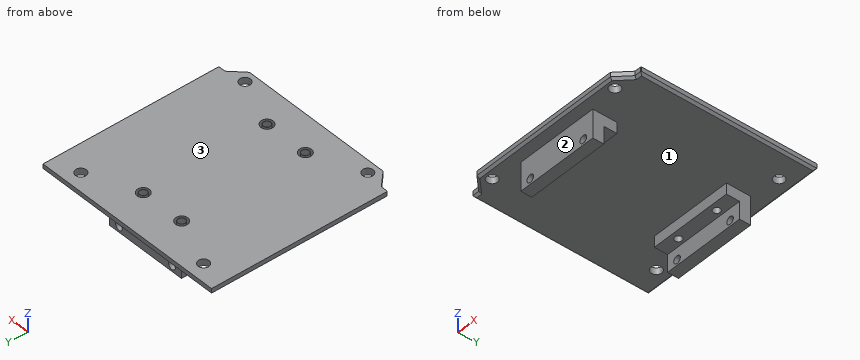
from build123d import *

# Parameters (mm, degrees)
SKETCH3_W             = 38
SKETCH3_H             = 6
BOSS_EXTRUDE2_DEPTH   = 8
BOSS_EXTRUDE2_2_DEPTH = 8
SKETCH1_R             = 2.43
BOSS_EXTRUDE3_DEPTH   = 3
CHAMFER1_SIZE         = 1
SKETCH4_W             = 38
SKETCH4_H             = 5
BOSS_EXTRUDE4_DEPTH   = 16
SKETCH5_R             = 1.75
CUT_EXTRUDE1_DEPTH    = 80
SKETCH6_R             = 1.625
CUT_EXTRUDE2_DEPTH    = 10
SKETCH7_R             = 2.75
SKETCH7_R_2           = 1.75
CUT_EXTRUDE3_DEPTH    = 4


with BuildPart() as part:
    # Sketch3 → Boss-Extrude2 (new body)
    with BuildSketch(Plane.XY):
        with Locations((152.499981225, 110.845805079)):
            Rectangle(SKETCH3_W, SKETCH3_H)
    extrude(amount=-BOSS_EXTRUDE2_DEPTH)



with BuildPart() as body_2:
    # Sketch3 → Boss-Extrude2 2 (new body)
    with BuildSketch(Plane.XY):
        with Locations((152.499981225, 166.845805079)):
            Rectangle(SKETCH3_W, SKETCH3_H)
    extrude(amount=-BOSS_EXTRUDE2_2_DEPTH)


with BuildPart() as body_3:
    # Sketch1 → Boss-Extrude3 (new body)
    with BuildSketch(Plane.XY):
        Polygon((197.000000954, 103.088447924), (197.000000954, 183.154169798), (107.999998748, 183.154169798), (107.999998748, 103.08845101), (108.242627497, 102.845828652), (111.242642284, 102.845828652), (117.242639543, 96.845823944), (187.757360159, 96.845823944), (193.757357418, 102.845828652), (196.757376569, 102.845828652), align=None)
        with Locations((184.906666899, 176.322621726)):
            Circle(SKETCH1_R, mode=Mode.SUBTRACT)
        with Locations((120.09, 176.322621726)):
            Circle(SKETCH1_R, mode=Mode.SUBTRACT)
        with Locations((184.906666899, 101.371103796)):
            Circle(SKETCH1_R, mode=Mode.SUBTRACT)
        with Locations((120.09, 101.371103796)):
            Circle(SKETCH1_R, mode=Mode.SUBTRACT)
    extrude(amount=-BOSS_EXTRUDE3_DEPTH)

    # Chamfer1
    # the kernel refuses this chamfer: 1 mm, written as the material it takes off along each edge
    with BuildSketch(Plane(origin=(105.670944509, 102.845828652, -3), x_dir=(0, -0.027495876610582174, 0.9996219169112968), z_dir=(1, 0, 0))) as chamfer1_piece_1_section:
        Polygon((CHAMFER1_SIZE * 0.999621916911, -CHAMFER1_SIZE * 0.0274958766106), (-CHAMFER1_SIZE * 0.0274958766106, -CHAMFER1_SIZE * 0.999621916911), (0, 0), align=None)
    chamfer1_piece_1 = extrude(amount=8.143380763, mode=Mode.PRIVATE)
    chamfer1_piece_1 = split(chamfer1_piece_1, bisect_by=Plane(origin=(109.611460338, 104.477012624, -2.663729969), z_dir=(-0.7071072202160112, -0.7071063421568112, 0)), keep=Keep.TOP, mode=Mode.PRIVATE)
    add(chamfer1_piece_1, mode=Mode.SUBTRACT)
    with BuildSketch(Plane(origin=(109.424188934, 104.664284261, -3), x_dir=(-0.019442532877514053, -0.01944250873450663, 0.9996219169112968), z_dir=(0.7071063421568113, -0.7071072202160114, 0))) as chamfer1_piece_2_section:
        Polygon((CHAMFER1_SIZE * 0.999621916911, -CHAMFER1_SIZE * 0.0274958766106), (-CHAMFER1_SIZE * 0.0274958766106, -CHAMFER1_SIZE * 0.999621916911), (0, 0), align=None)
    chamfer1_piece_2 = extrude(amount=13.628648741, mode=Mode.PRIVATE)
    chamfer1_piece_2 = split(chamfer1_piece_2, bisect_by=Plane(origin=(115.495387611, 102.845828652, -2.667041635), z_dir=(0, -1, 0)), keep=Keep.TOP, mode=Mode.PRIVATE)
    add(chamfer1_piece_2, mode=Mode.SUBTRACT)
    with BuildSketch(Plane(origin=(191.18567443, 102.845828652, -3), x_dir=(0, -0.027495876610582174, 0.9996219169112968), z_dir=(1, 0, 0))) as chamfer1_piece_3_section:
        Polygon((CHAMFER1_SIZE * 0.999621916911, -CHAMFER1_SIZE * 0.0274958766106), (-CHAMFER1_SIZE * 0.0274958766106, -CHAMFER1_SIZE * 0.999621916911), (0, 0), align=None)
    chamfer1_piece_3 = extrude(amount=8.143385128, mode=Mode.PRIVATE)
    chamfer1_piece_3 = split(chamfer1_piece_3, bisect_by=Plane(origin=(195.388540462, 104.477013723, -2.663729975), z_dir=(0.7071072202160112, -0.7071063421568112, 0)), keep=Keep.TOP, mode=Mode.PRIVATE)
    add(chamfer1_piece_3, mode=Mode.SUBTRACT)
    with BuildSketch(Plane(origin=(185.938906809, 95.027368335, -3), x_dir=(0.019442532877507145, -0.019442508734499722, 0.999621916911297), z_dir=(0.7071063421568113, 0.7071072202160114, 0))) as chamfer1_piece_4_section:
        Polygon((CHAMFER1_SIZE * 0.999621916911, -CHAMFER1_SIZE * 0.0274958766106), (-CHAMFER1_SIZE * 0.0274958766106, -CHAMFER1_SIZE * 0.999621916911), (0, 0), align=None)
    chamfer1_piece_4 = extrude(amount=13.628648741, mode=Mode.PRIVATE)
    chamfer1_piece_4 = split(chamfer1_piece_4, bisect_by=Plane(origin=(189.504612091, 102.845828652, -2.667041635), z_dir=(0, -1, 0)), keep=Keep.TOP, mode=Mode.PRIVATE)
    add(chamfer1_piece_4, mode=Mode.SUBTRACT)
    with BuildSketch(Plane(origin=(114.670956555, 96.845823944, -3), x_dir=(0, -0.027495876610582174, 0.9996219169112968), z_dir=(1, 0, 0))) as chamfer1_piece_5:
        Polygon((CHAMFER1_SIZE * 0.999621916911, -CHAMFER1_SIZE * 0.0274958766106), (-CHAMFER1_SIZE * 0.0274958766106, -CHAMFER1_SIZE * 0.999621916911), (0, 0), align=None)
    extrude(amount=75.658086593, mode=Mode.SUBTRACT)
    with BuildSketch(Plane(origin=(107.999998748, 185.725852786, -3), x_dir=(-0.027495876610582174, 0, 0.9996219169112968), z_dir=(0, -1, 0))) as chamfer1_piece_6:
        Polygon((CHAMFER1_SIZE * 0.999621916911, -CHAMFER1_SIZE * 0.0274958766106), (-CHAMFER1_SIZE * 0.0274958766106, -CHAMFER1_SIZE * 0.999621916911), (0, 0), align=None)
    extrude(amount=85.209084764, mode=Mode.SUBTRACT)
    with BuildSketch(Plane(origin=(199.571683942, 183.154169798, -3), x_dir=(0, 0.027495876610582174, 0.9996219169112968), z_dir=(-1, 0, 0))) as chamfer1_piece_7:
        Polygon((CHAMFER1_SIZE * 0.999621916911, -CHAMFER1_SIZE * 0.0274958766106), (-CHAMFER1_SIZE * 0.0274958766106, -CHAMFER1_SIZE * 0.999621916911), (0, 0), align=None)
    extrude(amount=94.143368181, mode=Mode.SUBTRACT)
    with BuildSketch(Plane(origin=(197.000000954, 100.516764936, -3), x_dir=(0.027495876610582174, 0, 0.9996219169112968), z_dir=(0, 1, 0))) as chamfer1_piece_8:
        Polygon((CHAMFER1_SIZE * 0.999621916911, -CHAMFER1_SIZE * 0.0274958766106), (-CHAMFER1_SIZE * 0.0274958766106, -CHAMFER1_SIZE * 0.999621916911), (0, 0), align=None)
    extrude(amount=85.20908785, mode=Mode.SUBTRACT)
    with BuildSketch(Plane(origin=(105.670944509, 102.845828652, -3), x_dir=(0, -0.027495876610582174, 0.9996219169112968), z_dir=(1, 0, 0))) as chamfer1_piece_9a_section:
        Polygon((CHAMFER1_SIZE * 0.999621916911, -CHAMFER1_SIZE * 0.0274958766106), (-CHAMFER1_SIZE * 0.0274958766106, -CHAMFER1_SIZE * 0.999621916911), (0, 0), align=None)
    chamfer1_piece_9a = extrude(amount=8.143380763, mode=Mode.PRIVATE)
    chamfer1_piece_9a = split(chamfer1_piece_9a, bisect_by=Plane(origin=(111.621802536, 102.46666793, -2.681906862), z_dir=(0.7071072202160112, 0.7071063421568112, 0)), keep=Keep.TOP, mode=Mode.PRIVATE)
    with BuildSketch(Plane(origin=(109.424188934, 104.664284261, -3), x_dir=(-0.019442532877514053, -0.01944250873450663, 0.9996219169112968), z_dir=(0.7071063421568113, -0.7071072202160114, 0))) as chamfer1_piece_9b_section:
        Polygon((CHAMFER1_SIZE * 0.999621916911, -CHAMFER1_SIZE * 0.0274958766106), (-CHAMFER1_SIZE * 0.0274958766106, -CHAMFER1_SIZE * 0.999621916911), (0, 0), align=None)
    chamfer1_piece_9b = extrude(amount=13.628648741, mode=Mode.PRIVATE)
    chamfer1_piece_9b = split(chamfer1_piece_9b, bisect_by=Plane(origin=(110.706428382, 102.845828652, -2.681906862), z_dir=(0, 1, 0)), keep=Keep.TOP, mode=Mode.PRIVATE)
    chamfer1_piece_9 = chamfer1_piece_9a & chamfer1_piece_9b
    add(chamfer1_piece_9, mode=Mode.SUBTRACT)
    with BuildSketch(Plane(origin=(185.938906809, 95.027368335, -3), x_dir=(0.019442532877507145, -0.019442508734499722, 0.999621916911297), z_dir=(0.7071063421568113, 0.7071072202160114, 0))) as chamfer1_piece_10a_section:
        Polygon((CHAMFER1_SIZE * 0.999621916911, -CHAMFER1_SIZE * 0.0274958766106), (-CHAMFER1_SIZE * 0.0274958766106, -CHAMFER1_SIZE * 0.999621916911), (0, 0), align=None)
    chamfer1_piece_10a = extrude(amount=13.628648741, mode=Mode.PRIVATE)
    chamfer1_piece_10a = split(chamfer1_piece_10a, bisect_by=Plane(origin=(194.29357132, 102.845828652, -2.681906862), z_dir=(0, 1, 0)), keep=Keep.TOP, mode=Mode.PRIVATE)
    with BuildSketch(Plane(origin=(191.18567443, 102.845828652, -3), x_dir=(0, -0.027495876610582174, 0.9996219169112968), z_dir=(1, 0, 0))) as chamfer1_piece_10b_section:
        Polygon((CHAMFER1_SIZE * 0.999621916911, -CHAMFER1_SIZE * 0.0274958766106), (-CHAMFER1_SIZE * 0.0274958766106, -CHAMFER1_SIZE * 0.999621916911), (0, 0), align=None)
    chamfer1_piece_10b = extrude(amount=8.143385128, mode=Mode.PRIVATE)
    chamfer1_piece_10b = split(chamfer1_piece_10b, bisect_by=Plane(origin=(193.378197166, 102.46666793, -2.681906862), z_dir=(-0.7071072202160112, 0.7071063421568112, 0)), keep=Keep.TOP, mode=Mode.PRIVATE)
    chamfer1_piece_10 = chamfer1_piece_10a & chamfer1_piece_10b
    add(chamfer1_piece_10, mode=Mode.SUBTRACT)


with BuildPart() as part_1:
    add(part.part)

    add(body_2.part)  # Boss-Extrude4 merges body 2

    add(body_3.part)  # Boss-Extrude4 merges body 3
    # Sketch4 → Boss-Extrude4 (add)
    with BuildSketch(Plane.XY):
        with Locations((152.499981225, 172.345805079)):
            Rectangle(SKETCH4_W, SKETCH4_H)
        with Locations((152.499981225, 105.345805079)):
            Rectangle(SKETCH4_W, SKETCH4_H)
    extrude(amount=-BOSS_EXTRUDE4_DEPTH)

    # Sketch5 → Cut-Extrude1 (cut)
    with BuildSketch(Plane(origin=(0, 102.845805079, 0), x_dir=(-1, 0, 0), z_dir=(0, -1, 0))):
        with Locations(Location((-166.499981225, 13.4, 0), (0, 0, 180))):
            Circle(SKETCH5_R)
        with Locations(Location((-138.499981225, 13.4, 0), (0, 0, 180))):
            Circle(SKETCH5_R)
    extrude(amount=-CUT_EXTRUDE1_DEPTH, mode=Mode.SUBTRACT)

    # Sketch6 → Cut-Extrude2 (cut)
    with BuildSketch(Plane(origin=(0, 0, -8), x_dir=(-1, 0, 0), z_dir=(0, 0, -1))):
        with Locations((-162.624981225, 110.595805079)):
            Circle(SKETCH6_R)
        with Locations((-142.374981225, 110.595805079)):
            Circle(SKETCH6_R)
        with Locations((-162.624981225, 167.095805079)):
            Circle(SKETCH6_R)
        with Locations((-142.374981225, 167.095805079)):
            Circle(SKETCH6_R)
    extrude(amount=-CUT_EXTRUDE2_DEPTH, mode=Mode.SUBTRACT)

    # Sketch7 → Cut-Extrude3 (cut)
    # profile 1 of 4: a face of its own
    with BuildSketch(Plane.XY):
        with Locations((162.624981225, 167.095805079)):
            Circle(SKETCH7_R)
        with Locations((162.624981225, 167.095805079)):
            Circle(SKETCH7_R_2, mode=Mode.SUBTRACT)
    # profile 2 of 4: a face of its own
    with BuildSketch(Plane.XY):
        with Locations((142.374981225, 167.095805079)):
            Circle(SKETCH7_R)
        with Locations((142.374981225, 167.095805079)):
            Circle(SKETCH7_R_2, mode=Mode.SUBTRACT)
    # profile 3 of 4: a face of its own
    with BuildSketch(Plane.XY):
        with Locations((162.624981225, 110.595805079)):
            Circle(SKETCH7_R)
        with Locations((162.624981225, 110.595805079)):
            Circle(SKETCH7_R_2, mode=Mode.SUBTRACT)
    # profile 4 of 4: a face of its own
    with BuildSketch(Plane.XY):
        with Locations((142.374981225, 110.595805079)):
            Circle(SKETCH7_R)
        with Locations((142.374981225, 110.595805079)):
            Circle(SKETCH7_R_2, mode=Mode.SUBTRACT)
    extrude(amount=-CUT_EXTRUDE3_DEPTH, mode=Mode.SUBTRACT)


solid = part_1.part
Check sheet for the modelled part. Datum: model origin and axes. Units: mm. Face numbers are marked on the shaded views. Coordinates: 2 decimals unless noted, no trailing zeros. Write each loop counter-clockwise with the first axis right and the second up, starting at its lowest first coordinate (ties: lowest second). Pieces come first, ordered by that corner, then holes.
Item 1: Scan lines: probe 1 along Y at (x, z) = (120.09, -1.9); probe 2 along Y at (x, z) = (168, -6.25); probe 3 along Y at (x, z) = (160, -12.5). Record each from-to range of solid material in increasing order.
Numbers:
probe 1: y = 96.85 to 98.94, 103.8 to 173.89, 178.75 to 183.15
probe 2: y = 102.85 to 113.85, 163.85 to 174.85
probe 3: y = 102.85 to 107.85, 169.85 to 174.85
Item 2: Depth check by flat-ended pin: pin 1 Ø4 at (x, y) = (120.09, 176.32) entering from +Z; pin 2 Ø3 at (x, y) = (150.5, 112.5) entering from -Z; pin 3 Ø1.5 at (x, z) = (161.5, -6.5) entering from +Y; pin 4 Ø5 at (x, y) = (162.62, 167.1) entering from +Z. Enter the tip coordinate at first touch or a pass-through.
Numbers:
pin 1: passes through
pin 2: stops at z = -8
pin 3: stops at y = 174.85
pin 4: stops at z = 0
Item 3: Cross-section at B-B on x = 120.09. Record the boundary of the cut face in (y, z), then the cut area to 3 significant figures.
Numbers:
outline: (96.85, -2) - (97.85, -3) - (98.94, -3) - (98.94, 0) - (96.85, 0) - close; (103.8, -3) - (173.89, -3) - (173.89, 0) - (103.8, 0) - close; (178.75, -3) - (182.15, -3) - (183.15, -2) - (183.15, 0) - (178.75, 0) - close
area: 229 mm2
Item 4: Cross-section at D-D on y = 136.5. Record the boundary of the cut face in (x, z), then the cut area to 3 significant figures.
Numbers:
outline: (108, -2) - (109, -3) - (196, -3) - (197, -2) - (197, 0) - (108, 0) - close
area: 266 mm2
Item 5: Mould release check, pull along Y, two halves, no side actions. Record for the marked faces 1, 2 and 3: released by +Y, released by -Y, zero draft, split by the parting line, or undercut.
Numbers:
face 1: undercut
face 2: released by -Y
face 3: zero draft
Item 6: Cross-section at A-A on z = -13.4. Record the boundary of the cut face in (x, y), then the cut area to 3 significant figures.
Numbers:
outline: (133.5, 102.85) - (136.75, 102.85) - (136.75, 107.85) - (133.5, 107.85) - close; (133.5, 169.85) - (136.75, 169.85) - (136.75, 174.85) - (133.5, 174.85) - close; (140.25, 102.85) - (164.75, 102.85) - (164.75, 107.85) - (140.25, 107.85) - close; (140.25, 169.85) - (164.75, 169.85) - (164.75, 174.85) - (140.25, 174.85) - close; (168.25, 102.85) - (171.5, 102.85) - (171.5, 107.85) - (168.25, 107.85) - close; (168.25, 169.85) - (171.5, 169.85) - (171.5, 174.85) - (168.25, 174.85) - close
area: 310 mm2
Item 7: Cross-section at C-C on z = -6. Record the boundary of the cut face in (x, y) (3 decimals), then the cut area to 3 significant figures.
Numbers:
outline: (133.5, 102.846) - (171.5, 102.846) - (171.5, 113.846) - (133.5, 113.846) - close; (133.5, 163.846) - (171.5, 163.846) - (171.5, 174.846) - (133.5, 174.846) - close; hole circle Ø3.25 at (142.375, 110.596); hole circle Ø3.25 at (142.375, 167.096); hole circle Ø3.25 at (162.625, 110.596); hole circle Ø3.25 at (162.625, 167.096)
area: 803 mm2
